Source: CAD feature listing. Evaluate the final solid. Frame: model axes, mm. Round coordinates to 2 decimals unless told otherwise and drop trailing zeros. Write each loop counter-clockwise with the first axis right and the second up, starting at its lowest first coordinate (ties: lowest second). Pieces come first, ordered by that corner, then holes.
from build123d import *

# Parameters (mm, degrees)
SKETCH1_R                                       = 27.5
BOSS_EXTRUDE1_DEPTH                             = 4
SKETCH2_R                                       = 40
BOSS_EXTRUDE2_DEPTH                             = 5
CIRPATTERN1_COUNT                               = 12
CSK_FOR_M4_FLAT_HEAD_MACHINE_SCREW2_D           = 4.5
CSK_FOR_M4_FLAT_HEAD_MACHINE_SCREW2_CSINK_D     = 9.4
CSK_FOR_M4_FLAT_HEAD_MACHINE_SCREW2_CSINK_ANGLE = 90
CIRPATTERN3_COUNT                               = 12
FILLET2_R                                       = 10


with BuildPart() as part:
    # Sketch1 → Boss-Extrude1 (new, symmetric)
    with BuildSketch(Plane.XY):
        Circle(SKETCH1_R)
    extrude(amount=BOSS_EXTRUDE1_DEPTH, both=True)

    # Sketch2 → Boss-Extrude2 (add)
    with BuildSketch(Plane.XY.offset(4)):
        Circle(SKETCH2_R)
    extrude(amount=BOSS_EXTRUDE2_DEPTH)

    # Sketch5 → M4x0.7 Tapped Hole1 (revolve, cut)
    with BuildSketch(Plane(origin=(0, 36.25, 9), x_dir=(0, -1, 0), z_dir=(1, 0, 0))):
        Polygon((0, 0), (0, 11.091420021), (1.65, 10.1), (1.65, 0.375), (2.025, 0), align=None)
    m4x0_7_tapped_hole1 = revolve(axis=Axis((0, 36.25, 15.35), (0, 0, -1)), mode=Mode.SUBTRACT)

    # CirPattern1: M4x0.7 Tapped Hole1 ×12 about axis
    cirpattern1_axis = Axis((0, -0.093143502, 0), (0, 0, 1))
    for i in range(1, CIRPATTERN1_COUNT):
        add(m4x0_7_tapped_hole1.rotate(cirpattern1_axis, i * 360 / CIRPATTERN1_COUNT), mode=Mode.SUBTRACT)

    # CSK for M4 Flat Head Machine Screw2 (through all)
    with Locations(Plane.XY.offset(9)):
        with Locations((21.733331092, 5.823428515)):
            csk_for_m4_flat_head_machine_screw2 = CounterSinkHole(CSK_FOR_M4_FLAT_HEAD_MACHINE_SCREW2_D / 2, CSK_FOR_M4_FLAT_HEAD_MACHINE_SCREW2_CSINK_D / 2, counter_sink_angle=CSK_FOR_M4_FLAT_HEAD_MACHINE_SCREW2_CSINK_ANGLE)

    # CirPattern3: CSK for M4 Flat Head Machine Screw2 ×12 about axis, 6 skipped
    cirpattern3_axis = Axis((-0.314050172, -0.081151288, 0), (0, 0, 1))
    add([csk_for_m4_flat_head_machine_screw2.rotate(cirpattern3_axis, i * 360 / CIRPATTERN3_COUNT) for i in range(1, CIRPATTERN3_COUNT) if i not in (2, 3, 6, 7, 10, 11)], mode=Mode.SUBTRACT)

    # Fillet2
    # the kernel refuses this fillet: 10 mm, written as the material it adds along each edge
    with BuildSketch(Plane(origin=(0, 0, 4), x_dir=(1, 0, 0), z_dir=(0, -1, 0))) as fillet2_piece_1_section:
        with BuildLine():
            CenterArc((37.297958971, -10), FILLET2_R, 90, 78.463040967)
            Line((37.297958971, 0), (37.297958971, 0.2))
            Line((37.297958971, 0.2), (27.5, 0.2))
            Line((27.5, 0.2), (27.3, 0))
            ThreePointArc((27.3, 0), (27.3, -4), (27.304040821, -7.96))
            Line((27.304040821, -7.96), (27.5, -8))
        make_face()
    fillet2_piece_1 = revolve(axis=Axis((0, 0, 4), (0, 0, 1)), mode=Mode.PRIVATE)
    fillet2_piece_1 = fillet2_piece_1 - Plane(origin=(18.171571751, 31.380942024, 1.87223315), x_dir=(-0.5000000000000004, -0.8660254037844384, 0), z_dir=(0, 0, 1)) * Cylinder(1.65, 150, mode=Mode.PRIVATE)
    fillet2_piece_1 = fillet2_piece_1 - Plane(origin=(31.474085526, 18.078428249, 1.87223315), x_dir=(-0.8660254037844386, -0.5000000000000001, 0), z_dir=(0, 0, 1)) * Cylinder(1.65, 150, mode=Mode.PRIVATE)
    fillet2_piece_1 = fillet2_piece_1 - Plane(origin=(36.343143502, -0.093143502, 1.87223315), x_dir=(-1, 0, 0), z_dir=(0, 0, 1)) * Cylinder(1.65, 150, mode=Mode.PRIVATE)
    fillet2_piece_1 = fillet2_piece_1 - Plane(origin=(0, 36.25, 1.87223315), x_dir=(0, -1, 0), z_dir=(0, 0, 1)) * Cylinder(1.65, 150, mode=Mode.PRIVATE)
    fillet2_piece_1 = fillet2_piece_1 - Plane(origin=(-18.171571751, 31.380942024, 1.87223315), x_dir=(0.49999999999999994, -0.8660254037844387, 0), z_dir=(0, 0, 1)) * Cylinder(1.65, 150, mode=Mode.PRIVATE)
    fillet2_piece_1 = fillet2_piece_1 - Plane(origin=(-31.474085526, 18.078428249, 1.87223315), x_dir=(0.8660254037844386, -0.5000000000000001, 0), z_dir=(0, 0, 1)) * Cylinder(1.65, 150, mode=Mode.PRIVATE)
    fillet2_piece_1 = fillet2_piece_1 - Plane(origin=(31.474085526, -18.264715253, 1.87223315), x_dir=(-0.8660254037844384, 0.5000000000000004, 0), z_dir=(0, 0, 1)) * Cylinder(1.65, 150, mode=Mode.PRIVATE)
    fillet2_piece_1 = fillet2_piece_1 - Plane(origin=(18.171571751, -31.567229028, 1.87223315), x_dir=(-0.5000000000000001, 0.8660254037844386, 0), z_dir=(0, 0, 1)) * Cylinder(1.65, 150, mode=Mode.PRIVATE)
    fillet2_piece_1 = fillet2_piece_1 - Plane(origin=(0, -36.436287004, 1.87223315), x_dir=(0, 1, 0), z_dir=(0, 0, 1)) * Cylinder(1.65, 150, mode=Mode.PRIVATE)
    fillet2_piece_1 = fillet2_piece_1 - Plane(origin=(-36.343143502, -0.093143502, 1.87223315), x_dir=(1, 0, 0), z_dir=(0, 0, 1)) * Cylinder(1.65, 150, mode=Mode.PRIVATE)
    fillet2_piece_1 = fillet2_piece_1 - Plane(origin=(-31.474085526, -18.264715253, 1.87223315), x_dir=(0.8660254037844388, 0.49999999999999983, 0), z_dir=(0, 0, 1)) * Cylinder(1.65, 150, mode=Mode.PRIVATE)
    fillet2_piece_1 = fillet2_piece_1 - Plane(origin=(-18.171571751, -31.567229028, 1.87223315), x_dir=(0.49999999999999994, 0.8660254037844388, 0), z_dir=(0, 0, 1)) * Cylinder(1.65, 150, mode=Mode.PRIVATE)
    add(fillet2_piece_1)


solid = part.part
1) Material intervals for line 1 (X direction, y = -33, z = 5); line 2 (X direction, y = -32.5, z = 5); line 3 (Y direction, x = -17.5, z = 8.25), sorted ascending.
Taken from the geometry:
line 1: x = -22.61 to -18.99, -17.35 to 17.35, 18.99 to 22.61
line 2: x = -23.32 to -19.53, -16.81 to 16.81, 19.53 to 23.32
line 3: y = -35.97 to -33.07, -30.06 to 12.25, 19.87 to 29.87, 32.89 to 35.97
2) Pull-direction query (X, two-part tool) for faces 1 (the face through (26.5, -26.5, 4)), 2 (the face through (18.2, 15.7, 6.7)), 3 (the face through (-8.67, -39.05, 6.46)); classes: released by +X, released by -X, zero draft, split by the parting line, or undercut.
Taken from the geometry:
face 1: zero draft
face 2: undercut
face 3: split by the parting line
3) Section query A-A on z = 2. Return the cut outline in (x, y).
Taken from the geometry:
outline: circle Ø62.6 at (0, 0); hole circle Ø4.5 at (-22.36, 5.83); hole circle Ø4.5 at (-16.45, 16.06); hole circle Ø4.5 at (-6.22, -22.13); hole circle Ø4.5 at (5.59, -22.13); hole circle Ø4.5 at (15.83, 16.06); hole circle Ø4.5 at (21.73, 5.82)
4) Contact query for flat-ended pins moving along their axis: P1, Ø2, axis at x = 24.5, z = 6.5, coming from the -Y side; P2, Ø5.5, axis at x = 0, y = -36.44, coming from the -Z side; P3, Ø4.5, axis at x = 18.17, y = 31.38, coming from the -Z side. Output: stop coordinate, or through.
Taken from the geometry:
P1: stops at y = -32.37
P2: stops at z = 3.33
P3: stops at z = 3.44
